Could you check a few things on this model? Use its own coordinates, in mm. A direction names the side the tool comes from. Give positions to 0.01 mm unless a question says otherwise; leave off trailing zeros. Order: outer loops, then holes, each group sorted by start corner. A loop starts at its lowest first (then second) coordinate and runs counter-clockwise, first axis right, second up. Notation, with made-up numbers: (74, -6.5) -> (112, -6.5) arc R24 ccw to (112, 23.5) -> close; hole circle Ø6 at (-5, 10.25). An arc over 180 degrees is marked (long way). One line per item, written item: value.
```python
from build123d import *

# Parameters (mm, degrees)
SKETCH_1_W          = 110
SKETCH_1_H          = 35
SKETCH_1_R          = 1.65
EXTRUDE_1_DEPTH     = 10
SKETCH_3_W          = 40
SKETCH_3_H          = 28
CUT_EXTRUDE_1_DEPTH = 4
FILLET_1_R          = 3
SKETCH_4_R          = 1.65
CUT_EXTRUDE_2_DEPTH = 66.954529791
CUT_EXTRUDE_3_DEPTH = 4
SKETCH_7_W          = 15
SKETCH_7_H          = 20
CUT_EXTRUDE_5_DEPTH = 59.576872569
CHAMFER_1_SIZE      = 1
SKETCH_8_R          = 10
CUT_EXTRUDE_6_DEPTH = 10


with BuildPart() as part:
    # 草图1 → 凸台-拉伸1 (new body)
    with BuildSketch(Plane.XY):
        Rectangle(SKETCH_1_W, SKETCH_1_H)
        with Locations((-17, 11)):
            Circle(SKETCH_1_R, mode=Mode.SUBTRACT)
        with Locations((17, 11)):
            Circle(SKETCH_1_R, mode=Mode.SUBTRACT)
        with Locations((17, -11)):
            Circle(SKETCH_1_R, mode=Mode.SUBTRACT)
        with Locations((-17, -11)):
            Circle(SKETCH_1_R, mode=Mode.SUBTRACT)
    extrude(amount=EXTRUDE_1_DEPTH)

    # 草图3 → 切除-拉伸1 (cut)
    with BuildSketch(Plane.XY.offset(10)):
        Rectangle(SKETCH_3_W, SKETCH_3_H)
    extrude(amount=-CUT_EXTRUDE_1_DEPTH, mode=Mode.SUBTRACT)

    # 圆角1
    fillet_1_edges = [part.edges().sort_by_distance(p)[0] for p in [
        (-20, -14, 8),
        (-20, 14, 8),
        (20, 14, 8),
        (20, -14, 8),
    ]]
    fillet(fillet_1_edges, radius=FILLET_1_R)

    # 草图4 → 切除-拉伸2 (cut, through all)
    with BuildSketch(Plane.XZ.offset(17.5)):
        with Locations((-51.5, 5)):
            Circle(SKETCH_4_R)
        with Locations(Location((51.5, 5, 0), (0, 0, 180))):
            Circle(SKETCH_4_R)
    extrude(amount=-CUT_EXTRUDE_2_DEPTH, mode=Mode.SUBTRACT)

    # 草图5 → 切除-拉伸3 (cut)
    with BuildSketch(Plane.XY.offset(6)):
        with BuildLine():
            Line((-17, -14.4), (17, -14.4))
            ThreePointArc((17, -14.4), (19.404163056, -13.404163056), (20.4, -11))
            Line((20.4, -11), (20.4, 11))
            ThreePointArc((20.4, 11), (19.404163056, 13.404163056), (17, 14.4))
            Line((17, 14.4), (-17, 14.4))
            ThreePointArc((-17, 14.4), (-19.404163056, 13.404163056), (-20.4, 11))
            Line((-20.4, 11), (-20.4, -11))
            ThreePointArc((-20.4, -11), (-19.404163056, -13.404163056), (-17, -14.4))
        make_face()
    extrude(amount=CUT_EXTRUDE_3_DEPTH, mode=Mode.SUBTRACT)

    # 草图7 → 切除-拉伸5 (cut, through all)
    with BuildSketch(Plane(origin=(0, 0, 0), x_dir=(-1, 0, 0), z_dir=(0, 0, -1))):
        with Locations((-55, 0)):
            Rectangle(SKETCH_7_W, SKETCH_7_H)
        with Locations((55, 0)):
            Rectangle(SKETCH_7_W, SKETCH_7_H)
    extrude(amount=-CUT_EXTRUDE_5_DEPTH, mode=Mode.SUBTRACT)

    # 倒角1
    chamfer_1_edges = [part.edges().sort_by_distance(p)[0] for p in [
        (55, -10, 5),
        (47.5, -10, 5),
        (55, 10, 5),
        (47.5, 10, 5),
        (-55, 10, 5),
        (-47.5, 10, 5),
        (-55, -10, 5),
        (-47.5, -10, 5),
    ]]
    chamfer(chamfer_1_edges, length=CHAMFER_1_SIZE)

    # 草图8 → 切除-拉伸6 (cut)
    with BuildSketch(Plane.XY.offset(6)):
        Circle(SKETCH_8_R)
    extrude(amount=-CUT_EXTRUDE_6_DEPTH, mode=Mode.SUBTRACT)


solid = part.part
```
1) Suppose I cut it at A-A, the plane x = 0. Write out the boundary of the cut face in (y, z).
Answer below:
outline: (-17.5, 0) -> (-10, 0) -> (-10, 6) -> (-14.4, 6) -> (-14.4, 10) -> (-17.5, 10) -> close; (10, 0) -> (17.5, 0) -> (17.5, 10) -> (14.4, 10) -> (14.4, 6) -> (10, 6) -> close
2) If I drill on line 1 along X through (y, z) = (11, 3.1); line 2 along Y through (x, z) = (17, 3.7); line 3 along X through (y, z) = (-3.5, 6.25), over which ranges is the centre line in solid material (lowest first)?
Answer below:
line 1: x = -55 to -18.65, -15.35 to 15.35, 18.65 to 55
line 2: y = -17.5 to -12.65, -9.35 to 9.35, 12.65 to 17.5
line 3: x = -47.5 to -20.4, 20.4 to 47.5
3) Suppose I cut it at B-B, the plane y = 0. Write out the boundary of the cut face in (x, z), then the cut area to 3 significant figures.
Answer below:
outline: (-47.5, 0) -> (-10, 0) -> (-10, 6) -> (-20.4, 6) -> (-20.4, 10) -> (-47.5, 10) -> close; (10, 0) -> (47.5, 0) -> (47.5, 10) -> (20.4, 10) -> (20.4, 6) -> (10, 6) -> close
area: 667 mm2
4) For faces 4 (the flat face through (-20.4, 0, 8)), 5 (the flat face through (-47.5, 0, 5)), 6 (the flat face through (50, 10, 4)), 7 (the cylindrical face through (-53.15, -13.8, 5.07)), 8 (the flat face through (55, 14, 5)), which set-ups out of +Z, -Z, +X, -X, +Y, -Y let a thin tool reach every point of the face, with its end or its side?
Answer below:
face 4: +Z
face 5: +Z, -Z, -X
face 6: +Z, -Z, +X
face 7: +Y, -Y
face 8: +Z, -Z, +X, +Y, -Y
5) Suppose I cut it at C-C, the plane x = -51.5. Write out the boundary of the cut face in (y, z).
Answer below:
outline: (-17.5, 0) -> (-10, 0) -> (-10, 3.35) -> (-17.5, 3.35) -> close; (-17.5, 6.65) -> (-10, 6.65) -> (-10, 10) -> (-17.5, 10) -> close; (10, 0) -> (17.5, 0) -> (17.5, 3.35) -> (10, 3.35) -> close; (10, 6.65) -> (17.5, 6.65) -> (17.5, 10) -> (10, 10) -> close
6) Suppose I cut it at D-D, the plane z = 8.75. Write out the boundary of the cut face in (x, y), then the cut area to 3 significant figures.
Answer below:
outline: (-55, -17.5) -> (55, -17.5) -> (55, -11) -> (54, -10) -> (48.5, -10) -> (47.5, -9) -> (47.5, 9) -> (48.5, 10) -> (54, 10) -> (55, 11) -> (55, 17.5) -> (-55, 17.5) -> (-55, 11) -> (-54, 10) -> (-48.5, 10) -> (-47.5, 9) -> (-47.5, -9) -> (-48.5, -10) -> (-54, -10) -> (-55, -11) -> close; hole (-20.4, -11) arc R3.4 ccw to (-17, -14.4) -> (17, -14.4) arc R3.4 ccw to (20.4, -11) -> (20.4, 11) arc R3.4 ccw to (17, 14.4) -> (-17, 14.4) arc R3.4 ccw to (-20.4, 11) -> close
area: 2,380 mm2
7) For P1, Ø4, axis at y = 6.5, z = 2, coming from the -X side; P2, Ø1, axis at y = 7.5, z = 5.5, coming from the +X side; P3, Ø5.5, axis at x = 17, y = -11, coming from the +Z side, each with a flat end and sliding along its axis, tell me the tip position at first contact or that it passes through.
Answer below:
P1: stops at x = -47.5
P2: stops at x = 47.5
P3: stops at z = 6
8) We'd pull the mould along Y, two halves only. Please class faces 1 (the cylindrical face through (18.524, 10.368, 2.958)), 2 (the flat face through (-1, 17.5, 5)), 3 (the cylindrical face through (53.15, 13.7, 4.93)): +Y half, -Y half, draft (parallel to the pull), parting line (faces both ways), or undercut.
Answer below:
face 1: undercut
face 2: +Y half
face 3: draft
